Read the model definition and answer for the solid it produces. Units are mm, in the model's axes. Face numbers are marked on the shaded views. Coordinates: 2 decimals unless noted, no trailing zeros. Write each loop counter-clockwise with the first axis right and the second up, starting at its lowest first coordinate (ties: lowest second). Pieces come first, ordered by that corner, then holes. Notation, with made-up numbers: M 54.25,-31 L 82.25,-31 A21 ccw 82.25,-23 Z; hole C 59,82.25 d7. An arc over 180 degrees is marked long. Use a Markdown table: item, result. Add a question column.
from build123d import *

# Parameters (mm, degrees)
F0_R     = 7.25
F1_DEPTH = 25.25
F3_R     = 11
F3_R_2   = 6.35
F4_DEPTH = 7.25


with BuildPart() as f1:
    # F0 (on Right) → F1 (new body, symmetric)
    with BuildSketch(Plane.YZ):
        with Locations((6.75, 0)):
            Circle(F0_R)
    extrude(amount=F1_DEPTH, both=True)

    # F2: F1 across plane


with BuildPart() as f1_1:
    add(f1.part)
    add(f1.part.mirror(Plane.XZ))


with BuildPart() as f4:
    # F3 (on Top) → F4 (new body, symmetric)
    with BuildSketch(Plane.XY):
        Circle(F3_R)
        Circle(F3_R_2, mode=Mode.SUBTRACT)
    extrude(amount=F4_DEPTH, both=True)


solid = f1_1.part
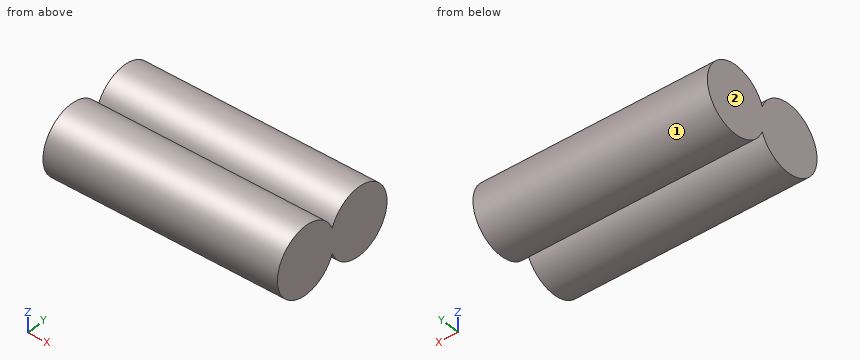
Item 1: Consider probe 1 along Y at (x, z) = (22, -3.75); probe 2 along Y at (x, z) = (9, -3); probe 3 along Z at (x, y) = (16, -6.5). Determine where each line is inside the solid, lowest interval first.
Item 2: Each of these flat-tipped pins is pushed along its axis until it touches: pin 1 (6 mm diameter, centred on x = -5.5, z = 5, fed in from -Y); pin 2 (1.5 mm diameter, centred on x = 9, y = 5, fed in from -Z); pin 3 (1 mm diameter, centred on x = -15, y = -8.5, fed in from +Z). Where does it stop, or does it pass through?
Item 3: Find section C-C on x = 20.5. Give the vertices of the cut face in (y, z).
Item 4: Find section A-A on z = 5.25. Give the vertices of the cut face in (x, y), then the cut area to 3 significant figures.
Item 5: Find section B-B on z = -5. Give the vertices of the cut face in (x, y).
Item 6: Determine the mould class of the marked faces 1 and 2 for opening direction Y: pulls with the +Y half, pulls with the -Y half, needs draft (parallel to the pull), parting line crosses it, or undercut.
Geometry says:
| question | item | result |
|---|---|---|
| 1 | probe 1 | y = -12.95 to -0.55, 0.55 to 12.95 |
| 1 | probe 2 | y = -13.35 to -0.15, 0.15 to 13.35 |
| 1 | probe 3 | z = -7.25 to 7.25 |
| 2 | pin 1 | stops at y = -13.72 |
| 2 | pin 2 | stops at z = -7.18 |
| 2 | pin 3 | stops at z = 7.14 |
| 3 | outline | M 0,-2.65 A7.25 ccw long 0,2.65 A7.25 ccw long Z |
| 4 | outline | M -25.25,-11.75 L 25.25,-11.75 L 25.25,-1.75 L -25.25,-1.75 Z; M -25.25,1.75 L 25.25,1.75 L 25.25,11.75 L -25.25,11.75 Z |
| 4 | area | 1,010 mm2 |
| 5 | outline | M -25.25,-12 L 25.25,-12 L 25.25,-1.5 L -25.25,-1.5 Z; M -25.25,1.5 L 25.25,1.5 L 25.25,12 L -25.25,12 Z |
| 6 | face 1 | undercut |
| 6 | face 2 | needs draft |
